from build123d import *

# Parameters (mm, degrees)
F0_R     = 3.5
F1_DEPTH = 10
F2_T     = -1.5


# Not quite as in the source:
# - a fillet or chamfer that OpenCascade refuses, or shapes differently, is made with other operations: its cross-section is extruded or revolved along the edge and cut away or added


with BuildPart() as f1:
    # F0 (on Top) → F1 (new body)
    with BuildSketch(Plane.XY):
        with Locations((-2.5134360774, -2.4357009433)):
            Circle(F0_R)
    extrude(amount=F1_DEPTH)

    # F2
    f2_openings = [f1.faces().sort_by_distance(p)[0] for p in [
        (-2.513436, -2.435701, 0),
    ]]
    offset(amount=F2_T, openings=f2_openings)

    # F3: chamfer of 5 on 1 edges, made by hand

    # F3_s1 → F3_t2 (revolve, cut)
    with BuildSketch(Plane.XZ.offset(2.4357009433)):
        Polygon((4.4865639226, 0), (-0.5134360774, 5), (-0.5134360774, 0), align=None)
    revolve(axis=Axis((-2.5134360774, -2.4357009433, 0), (0, 0, 1)), mode=Mode.SUBTRACT)


solid = f1.part
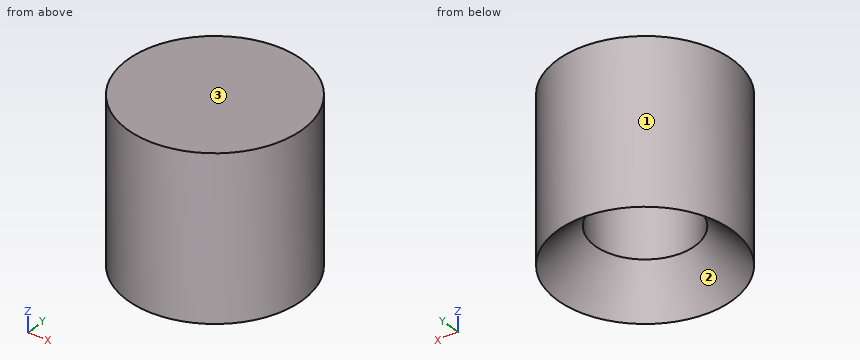
The listing builds one solid part. Answer for the finished solid, in the listing's coordinates (mm). Face numbers are marked on the shaded views. Round coordinates to 2 decimals unless told otherwise and drop trailing zeros. Write each loop counter-clockwise with the first axis right and the second up, starting at its lowest first coordinate (ties: lowest second). Pieces come first, ordered by that corner, then holes. Notation, with made-up numbers: (55.5, 49) - (90.5, 49) arc R30 cw to (90.5, 83) - close; hole circle Ø2 at (84.25, 16). An arc over 180 degrees is marked (long way). Use one line per item in the form item = value. Start each with the question number.
Item 1: Determine the mould class of the marked faces 1, 2 and 3 for opening direction X: +X half, -X half, draft (parallel to the pull), parting line (faces both ways), or undercut.
Item 2: Find the intervals of material crossed by line 1 (Z direction, x = -2, y = -4.25); line 2 (X direction, y = -1.5, z = 5.75); line 3 (Y direction, x = -4, z = 6.5), in increasing order. Write a range as [from, to].
Item 3: A cutting plane is placed at A-A (z = 8). Write down the section's boundary in (x, y).
Item 4: Flat-ended cylindrical pins translate along their axes: pin 1 Ø1 at (y, z) = (-4, 7.5) entering from +X; pin 2 Ø1 at (x, y) = (-2, 0) entering from -Z. Find the tip coordinate at first contact, or state that the pin passes through.
Item 5: A cutting plane is placed at B-B (z = 8.75). Write down the section's boundary in (x, y), plus the area to 3 significant figures.
The answers:
q1.face_1 = parting line
q1.face_2 = undercut
q1.face_3 = draft
q2.line_1 = [8.5, 10]
q2.line_2 = [-5.89, -4.28], [-0.75, 0.86]
q2.line_3 = [-5.6, -3.77], [-1.1, 0.73]
q3.outline = circle Ø7 at (-2.51, -2.44); hole circle Ø4 at (-2.51, -2.44)
q4.pin_1 = 0.82
q4.pin_2 = 4.01
q5.outline = circle Ø7 at (-2.51, -2.44)
q5.area = 38.5 mm^2
